Part model, mm, in its own coordinate system. A direction names the side the tool comes from. Give positions to 0.01 mm unless a question says otherwise; leave off trailing zeros. Order: outer loops, then holes, each group sorted by start corner. A loop starts at its lowest first (then second) coordinate and runs counter-clockwise, first axis right, second up. Notation, with made-up numbers: (41.25, -2.75) - (73.25, -2.75) arc R16 ccw to (73.25, 20.25) - close; hole circle Ø8 at (-10.75, 88.25). An arc over 180 degrees is marked (long way). One line per item, written item: value.
Autodesk Inventor part; units mm, degrees
ref_plane "Work Plane1" through (0, 0, 50) normal (0, 0, 1) x (1, 0, 0)
ref_plane "Work Plane2" through (15, 0, 0) normal (1, 0, 0) x (0, 1, 0)
ref_plane "XZ Plane" through (0, 0, 0) normal (0, 1, 0) x (-1, 0, 0)
sketch "Sketch1" plane through (0, 0, 0) normal (0, 0, 1) x (1, 0, 0)
  line L0 (0, 0) -> (30, 0)
  line L1 (30, 0) -> (30, 65)
  line L2 (30, 65) -> (0, 65)
  line L3 (0, 65) -> (0, 0)
  dimension "d0" = 30
  dimension "d1" = 65
extrude "Extrusion1" add sketch "Sketch1" along normal blind 100
sketch "Sketch2" plane through (0, 0, 100) normal (0, 0, 1) x (1, 0, 0)
  line L0 (2.1, 2.877) -> (27.9, 2.877)
  line L1 (27.9, 2.877) -> (27.9, 68.621)
  line L2 (27.9, 68.621) -> (2.1, 68.621)
  line L3 (2.1, 68.621) -> (2.1, 2.877)
  line L4 (30, 65) -> (0, 65) construction
  line L5 (15, 65) -> (15, 0) construction
  line L6 (0, 0) -> (30, 0) construction
  dimension "d4" = 25.8
extrude "Extrusion2" cut sketch "Sketch2" against normal blind 100
ref_plane "Work Plane1" through (0, 0, 50) normal (0, 0, 1) x (1, 0, 0)
sketch "Sketch3" plane through (0, 0, 50) normal (0, 0, 1) x (1, 0, 0)
  line L0 (2.1, 2.877) -> (27.9, 2.877) construction
  line L1 (15, 2.877) -> (15, 72.0179) construction
  line L2 (15, 65) -> (2.1, 65) construction
  line L3 (2.1, 65) -> (0, 65) construction
  line L4 (2.1, 65) -> (2.6, 65)
  line L5 (2.6, 65) -> (2.6, 60)
  line L6 (2.6, 60) -> (2.1, 60)
  line L7 (2.1, 60) -> (2.1, 65)
  line L8 (15, 60) -> (5.475, 60) construction
  line L9 (5.475, 60) -> (2.1, 60)
  line L10 (2.1, 60) -> (2.1, 2.877)
  line L11 (2.1, 2.877) -> (5.475, 2.877)
  line L12 (5.475, 2.877) -> (5.475, 60)
  point P0 (0, 0)
  dimension "d8" = 0.5
  dimension "d9" = 5
  dimension "d10" = 9.525
extrude "Extrusion3" add sketch "Sketch3" along normal mid plane 99
ref_plane "Work Plane2" through (15, 0, 0) normal (1, 0, 0) x (0, 1, 0)
mirror "Mirror1" about plane through (15, 0, 0) normal (1, 0, 0) of "Extrusion3"
split "Split1" plane through (0, 0, 50) removes the side toward (0, 0, -1)
sketch "Sketch4" plane through (30, 0, 50) normal (0, 0, -1) x (-1, 0, 0)
  line L0 (27.9, 2.877) -> (27.9, 65)
  line L1 (2.1, 65) -> (2.1, 2.877)
  line L2 (27.9, 2.877) -> (2.1, 2.877)
  line L3 (2.1, 2.877) -> (2.1, 65)
  line L4 (2.1, 65) -> (27.9, 65)
  line L5 (27.9, 65) -> (27.9, 2.877)
  point P0 (30, 0)
extrude "Extrusion4" cut sketch "Sketch4" against normal blind 0.5
properties part number "Reactor Bottom_v2" material "Polyethylene, Low Density"
1) Two-plate mould, pull along X, no slides. Class faces 5 (the face through (2.6, 63, 75)), 6 (the face through (30, 32, 75)), 7 (the face through (28.3, 27.8, 50)): pulls with the +X half, pulls with the -X half, needs draft (parallel to the pull), parting line crosses it, or undercut.
Answer:
face 5: undercut
face 6: pulls with the +X half
face 7: needs draft
2) Slice it at C-C on x = 26.5. Write the cut outline in (y, z).
Answer:
outline: (0, 50) - (2.88, 50) - (2.88, 50.5) - (60, 50.5) - (60, 99.5) - (2.88, 99.5) - (2.88, 100) - (0, 100) - close
3) Wall check: line 1 along X through (y, z) = (25, 57.5) (3 decimals); line 2 along Y through (x, z) = (3.5, 77); line 3 along Y through (x, z) = (20.75, 93.5). Give the ranges that are in metal, low to high. Write a range as [from, to].
Answer:
line 1: x = [0, 5.475], [24.525, 30]
line 2: y = [0, 60]
line 3: y = [0, 2.88]
4) Which spindle directions (+Z, -Z, +X, -X, +Y, -Y) get a long thin tool onto all of the face, cutting with end or side? Do faces 1 (the face through (26, 34, 50.5)), 2 (the face through (29, 65, 75)), 3 (the face through (24.525, 32, 75)), 4 (the face through (26, 34, 99.5)). Say none if no direction does.
Answer:
face 1: -Z, +Y
face 2: +Z, -Z, +X, -X, +Y
face 3: +Z, -Z, +Y
face 4: +Z, +Y
5) Drop flat-ended pins along their axis: P1, Ø2.5, axis at x = 26, y = 34.5, coming from the +Z side; P2, Ø1, axis at x = 9.5, z = 64.5, coming from the +Y side; P3, Ø2, axis at x = 24, y = 42.5, coming from the -Z side. Give the stop position or say it passes through.
Answer:
P1: stops at z = 99.5
P2: stops at y = 2.88
P3: stops at z = 50.5
6) Slice it at D-D on x = 8.75. Write the cut outline in (y, z).
Answer:
outline: (0, 50) - (2.88, 50) - (2.88, 100) - (0, 100) - close
7) Slice it at B-B on z = 74. Write the cut outline in (x, y) (3 decimals), then the cut area to 3 significant figures.
Answer:
outline: (0, 0) - (30, 0) - (30, 65) - (27.4, 65) - (27.4, 60) - (24.525, 60) - (24.525, 2.877) - (5.475, 2.877) - (5.475, 60) - (2.6, 60) - (2.6, 65) - (0, 65) - close
area: 738 mm2
8) Slice it at A-A on y = 39.5. Write the cut outline in (x, z) (3 decimals), then the cut area to 3 significant figures.
Answer:
outline: (0, 50) - (2.1, 50) - (2.1, 50.5) - (5.475, 50.5) - (5.475, 99.5) - (2.1, 99.5) - (2.1, 100) - (0, 100) - close; (24.525, 50.5) - (27.9, 50.5) - (27.9, 50) - (30, 50) - (30, 100) - (27.9, 100) - (27.9, 99.5) - (24.525, 99.5) - close
area: 541 mm2
